```python
from build123d import *

# Parameters (mm, degrees)
CROQUIS1_R              = 11.5
CROQUIS1_R_2            = 4.35
CROQUIS1_R_3            = 1.7000000000000004
SALIENTE_EXTRUIR1_DEPTH = 3.5
CROQUIS2_R              = 5.35
CROQUIS2_R_2            = 4.35
SALIENTE_EXTRUIR2_DEPTH = 14
CORTAR_EXTRUIR1_START   = -5
CORTAR_EXTRUIR1_DEPTH   = 5
CROQUIS4_R              = 5.275
CROQUIS4_R_2            = 4.35
CORTAR_EXTRUIR2_DEPTH   = 2
REDONDEO1_R             = 0.6
REDONDEO2_R             = 0.5
SALIENTE_EXTRUIR3_DEPTH = 3.5


with BuildPart() as part:
    # Croquis1 → Saliente-Extruir1 (new body)
    with BuildSketch(Plane(origin=(0, 0, 0), x_dir=(1, 0, 0), z_dir=(0, 1, 0))):
        with Locations(Location((1.731948e-11, 0, 0), (0, 0, 270))):
            Circle(CROQUIS1_R)
        with Locations(Location((1.731948e-11, 0, 0), (0, 0, 270))):
            Circle(CROQUIS1_R_2, mode=Mode.SUBTRACT)
        with Locations(Location((5.656854249492441, 5.65685424949238, 0), (0, 0, 270))):
            Circle(CROQUIS1_R_3, mode=Mode.SUBTRACT)
        with Locations(Location((-5.656854249492318, 5.656854249492381, 0), (0, 0, 270))):
            Circle(CROQUIS1_R_3, mode=Mode.SUBTRACT)
        with Locations(Location((-5.656854249492318, -5.656854249492381, 0), (0, 0, 270))):
            Circle(CROQUIS1_R_3, mode=Mode.SUBTRACT)
        with Locations(Location((5.656854249492441, -5.65685424949238, 0), (0, 0, 270))):
            Circle(CROQUIS1_R_3, mode=Mode.SUBTRACT)
    extrude(amount=SALIENTE_EXTRUIR1_DEPTH)

    # Croquis2 → Saliente-Extruir2 (add)
    with BuildSketch(Plane(origin=(0, 3.5, 0), x_dir=(1, 0, 0), z_dir=(0, 1, 0))):
        with Locations(Location((1.731948e-11, 0, 0), (0, 0, 270))):
            Circle(CROQUIS2_R)
        with Locations(Location((1.731948e-11, 0, 0), (0, 0, 270))):
            Circle(CROQUIS2_R_2, mode=Mode.SUBTRACT)
    extrude(amount=SALIENTE_EXTRUIR2_DEPTH)

    # Croquis3 → Cortar-Extruir1 (cut)
    with BuildSketch(Plane(origin=(0, 17.5, 0), x_dir=(1, 0, 0), z_dir=(0, 1, 0)).offset(CORTAR_EXTRUIR1_START)):
        with BuildLine():
            Line((1.732086e-11, 5.35), (1.732072e-11, 4.35))
            ThreePointArc((1.732072e-11, 4.35), (3.0759144981543076, 3.0759144981369877), (4.34999999998268, 0))
            Line((4.34999999998268, 0), (5.34999999998268, 0))
            ThreePointArc((5.34999999998268, 0), (3.783021279340855, 3.783021279323535), (1.732086e-11, 5.35))
        make_face()
        with BuildLine():
            Line((1.732086e-11, -5.35), (1.732072e-11, -4.35))
            ThreePointArc((1.732072e-11, -4.35), (-3.075914498144163, -3.075914498161481), (-4.34999999998268, 0))
            Line((-4.34999999998268, 0), (-5.34999999998268, 0))
            ThreePointArc((-5.34999999998268, 0), (-3.7830212793307103, -3.7830212793480285), (1.732086e-11, -5.35))
        make_face()
    extrude(amount=CORTAR_EXTRUIR1_DEPTH, mode=Mode.SUBTRACT)

    # Croquis4 → Cortar-Extruir2 (cut)
    with BuildSketch(Plane.XZ):
        with Locations(Location((1.731948e-11, 0, 0), (0, 0, 270))):
            Circle(CROQUIS4_R)
        with Locations(Location((1.731948e-11, 0, 0), (0, 0, 270))):
            Circle(CROQUIS4_R_2, mode=Mode.SUBTRACT)
    extrude(amount=-CORTAR_EXTRUIR2_DEPTH, mode=Mode.SUBTRACT)

    # Redondeo1
    redondeo1_edges = [part.edges().sort_by_distance(p)[0] for p in [
        (1.732109e-11, 0, 5.275),
    ]]
    fillet(redondeo1_edges, radius=REDONDEO1_R)

    # Redondeo2
    # the kernel refuses this fillet: 0.5 mm, written as the material it takes off along each edge
    with BuildSketch(Plane(origin=(-4.34999999998268, 12.5, -2.1e-16), x_dir=(0.05161519234821224, 0, -0.9986670475783493), z_dir=(0, 1, 0))) as redondeo2_piece_1:
        with BuildLine():
            CenterArc((0.4748597696035476, 0.49933352378917434), REDONDEO2_R, 182.9586473758917, 84.08270524821648)
            Line((-0.02447375418562714, 0.4735259276150691), (0, 0))
            ThreePointArc((0, 0), (0.22452608671472166, 0.00579834303418057), (0.44905217342944187, 0))
        make_face()
    extrude(amount=6.185394894032285, mode=Mode.SUBTRACT)
    with BuildSketch(Plane(origin=(-5.34999999998268, 12.5, 0), x_dir=(1, 0, 0), z_dir=(0, 1, 0))) as redondeo2_piece_2:
        with BuildLine():
            CenterArc((0.5258420423870858, 0.5), REDONDEO2_R, 174.08270524821654, 95.91729475178346)
            ThreePointArc((0.02850617046822812, 0.5515463917525764), (0.00713129545583069, 0.27614127906293384), (0, 0))
            Line((0, 0), (0.5258420423870858, 0))
        make_face()
    extrude(amount=6.3807063953146645, mode=Mode.SUBTRACT)
    with BuildSketch(Plane(origin=(1.73185e-11, 12.5, 5.35), x_dir=(4.4e-15, 0, -1), z_dir=(0, 1, 0))) as redondeo2_piece_3:
        with BuildLine():
            CenterArc((0.5258420423870889, -0.5), REDONDEO2_R, 90.00000000000026, 95.91729475178363)
            ThreePointArc((0.02850617046823233, -0.5515463917525796), (0.0071312954558319, -0.27614127906293445), (0, 0))
            Line((0, 0), (0.5258420423870867, 0))
        make_face()
    extrude(amount=6.380706395314672, mode=Mode.SUBTRACT)
    with BuildSketch(Plane(origin=(1.731868e-11, 12.5, 4.35), x_dir=(0.9986670475783493, 0, -0.051615192348211894), z_dir=(0, 1, 0))) as redondeo2_piece_4:
        with BuildLine():
            CenterArc((0.474859769603551, -0.49933352378917434), REDONDEO2_R, 92.95864737589183, 84.08270524821639)
            Line((-0.0244737541856237, -0.4735259276150684), (0, 0))
            ThreePointArc((0, 0), (0.2245260867147224, -0.00579834303418053), (0.4490521734294448, 0))
        make_face()
    extrude(amount=6.185394894032285, mode=Mode.SUBTRACT)
    with BuildSketch(Plane(origin=(1.732072e-11, 12.5, -4.35), x_dir=(-0.9986670475783493, 0, 0.05161519234821218), z_dir=(0, 1, 0))) as redondeo2_piece_5:
        with BuildLine():
            CenterArc((0.474859769603548, -0.49933352378917434), REDONDEO2_R, 92.95864737589177, 84.08270524821641)
            Line((-0.02447375418562666, -0.47352592761506823), (0, 0))
            ThreePointArc((0, 0), (0.22452608671472019, -0.00579834303418048), (0.4490521734294423, 0))
        make_face()
    extrude(amount=6.185394894032285, mode=Mode.SUBTRACT)
    with BuildSketch(Plane(origin=(1.732103e-11, 12.5, -5.35), x_dir=(-4.2e-16, 0, 1), z_dir=(0, 1, 0))) as redondeo2_piece_6:
        with BuildLine():
            CenterArc((0.525842042387086, -0.5), REDONDEO2_R, 90.00000000000003, 95.91729475178352)
            ThreePointArc((0.02850617046822835, -0.5515463917525767), (0.00713129545583081, -0.27614127906293173), (0, 0))
            Line((0, 0), (0.5258420423870858, 0))
        make_face()
    extrude(amount=6.3807063953146645, mode=Mode.SUBTRACT)
    with BuildSketch(Plane(origin=(4.34999999998268, 12.5, 1.9e-16), x_dir=(-0.05161519227127975, 0, 0.9986670475823255), z_dir=(0, 1, 0))) as redondeo2_piece_7:
        with BuildLine():
            CenterArc((0.47485976964022647, 0.4993335237871862), REDONDEO2_R, 182.95864737147792, 84.08270524821648)
            Line((-0.02447375415093636, 0.4735259276515472), (0, 0))
            ThreePointArc((0, 0), (0.22452608671427532, 0.00579834305147695), (0.44905217342765447, 0))
        make_face()
    extrude(amount=6.1853948941188825, mode=Mode.SUBTRACT)
    with BuildSketch(Plane(origin=(5.34999999998268, 12.5, 0), x_dir=(-1, 0, 0), z_dir=(0, 1, 0))) as redondeo2_piece_8:
        with BuildLine():
            CenterArc((0.5258420423524468, 0.5), REDONDEO2_R, 174.08270524821646, 95.91729475178352)
            ThreePointArc((0.02850617043359005, 0.5515463917525769), (0.0071312954212388, 0.2761412790638265), (0, 0))
            Line((0, 0), (0.5258420423524468, 0))
        make_face()
    extrude(amount=6.380706395310195, mode=Mode.SUBTRACT)

    # Croquis5 → Saliente-Extruir3 (add)
    with BuildSketch(Plane(origin=(0, 3.5, 0), x_dir=(1, 0, 0), z_dir=(0, 1, 0))):
        with BuildLine():
            Line((-4.867801495370659, 2.219686599837588), (-10.46349854147086, 4.7712889529219185))
            ThreePointArc((-10.46349854147086, 4.7712889529219185), (-11.49999999998268, 1.41e-15), (-10.46349854147086, -4.771288952921916))
            Line((-10.46349854147086, -4.771288952921914), (-4.86780149537066, -2.219686599837586))
            ThreePointArc((-4.86780149537066, -2.219686599837586), (-5.34999999998268, 8.9e-16), (-4.86780149537066, 2.219686599837588))
        make_face()
        with BuildLine():
            Line((-2.2196865998351183, -4.867801495381207), (-4.77128895293652, -10.463498541473625))
            ThreePointArc((-4.771288952936522, -10.463498541473623), (-6.77758e-12, -11.5), (4.771288952927311, -10.463498541493617))
            Line((4.771288952927309, -10.46349854149362), (2.2196865998493576, -4.86780149539051))
            ThreePointArc((2.219686599849358, -4.867801495390509), (6.10956e-12, -5.35), (-2.219686599835118, -4.867801495381206))
        make_face()
        with BuildLine():
            ThreePointArc((11.50000000001732, 0), (11.237887551221265, 2.4412872396535783), (10.463498541496383, 4.771288952941911))
            Line((10.463498541496381, 4.7712889529419105), (4.867801495401058, 2.2196865998468893))
            ThreePointArc((4.867801495401059, 2.2196865998468898), (5.228060730360026, 1.1357292810562294), (5.350000000017321, -1.1e-16))
            ThreePointArc((5.350000000017321, -1.1e-16), (5.228060730360026, -1.1357292810562303), (4.867801495401057, -2.2196865998468898))
            Line((4.867801495401058, -2.2196865998468898), (10.463498541496381, -4.771288952941912))
            ThreePointArc((10.463498541496378, -4.7712889529419185), (11.237887551221265, -2.4412872396535787), (11.50000000001732, -2.82e-15))
        make_face()
        with BuildLine():
            ThreePointArc((4.771288952927309, 10.46349854149362), (-6.77732e-12, 11.5), (-4.771288952936519, 10.463498541473625))
            Line((-4.771288952936519, 10.463498541473623), (-2.2196865998351187, 4.867801495381207))
            ThreePointArc((-2.219686599835118, 4.867801495381207), (6.10867e-12, 5.35), (2.219686599849357, 4.86780149539051))
            Line((2.2196865998493576, 4.86780149539051), (4.771288952927309, 10.46349854149362))
        make_face()
    extrude(amount=SALIENTE_EXTRUIR3_DEPTH)


solid = part.part
```
Build history of the part. All positions in model axes, mm. A direction names the side the tool comes from. Coordinates: 2 decimals unless noted, no trailing zeros. Order: outer loops, then holes, each group sorted by start corner. A loop starts at its lowest first (then second) coordinate and runs counter-clockwise, first axis right, second up.
Item 1: Drill centre lines: L1, parallel to Y at x = 9.5, z = 1.5; L2, parallel to Y at x = 2, z = -4.75; L3, parallel to X at y = 5.5, z = -1.5. Where is each one in solid material? Low to high.
Filled in:
L1: y = 0 to 7
L2: y = 2 to 12.5
L3: x = -11.4 to -4.08, 4.08 to 11.4
Item 2: Mould opens along X. For faces 1 (the flat face through (3.51, 5.23, 7.7)), 2 (the flat face through (7, 3.5, -7)), 3 (the flat face through (-8, 0, 0)) say: released by +X, released by -X, zero draft, split by the parting line, or undercut.
Filled in:
face 1: released by +X
face 2: undercut
face 3: zero draft
Item 3: Saw through at B-B on x = 9.75. List the corners of the cut face in (y, z).
Filled in:
outline: (0, -6.1) - (3.5, -6.1) - (3.5, -4.45) - (7, -4.45) - (7, 4.45) - (3.5, 4.45) - (3.5, 6.1) - (0, 6.1) - close
Item 4: Drop flat-ended pins along their axis: pin 1 Ø5 at (x, y) = (2.5, 15) entering from +Z; pin 2 Ø2 at (x, z) = (-2.5, 7) entering from +Y; pin 3 Ø8.5 at (x, z) = (-1, -1) entering from -Y. Give the stop position or say it passes through.
Filled in:
pin 1: stops at z = 5.32
pin 2: stops at y = 7
pin 3: stops at y = 0.04
Item 5: Saw through at C-C on z = 9.5. List the corners of the cut face in (x, y), then the cut area to 3 significant figures.
Filled in:
outline: (-6.48, 0) - (6.48, 0) - (6.48, 3.5) - (4.33, 3.5) - (4.33, 7) - (-4.33, 7) - (-4.33, 3.5) - (-6.48, 3.5) - close
area: 75.7 mm2
Item 6: Saw through at D-D on y = 2.5. List the corners of the cut face in (x, z).
Filled in:
outline: circle Ø23 at (0, 0); hole circle Ø3.4 at (-5.66, -5.66); hole circle Ø3.4 at (-5.66, 5.66); hole circle Ø8.7 at (0, 0); hole circle Ø3.4 at (5.66, -5.66); hole circle Ø3.4 at (5.66, 5.66)
Item 7: Saw through at A-A on y = 6. List the corners of the cut face in (x, z).
Filled in:
outline: (-10.46, -4.77) - (-4.87, -2.22) arc R5.35 ccw to (-2.22, -4.87) - (-4.77, -10.46) arc R11.5 ccw to (4.77, -10.46) - (2.22, -4.87) arc R5.35 ccw to (4.87, -2.22) - (10.46, -4.77) arc R11.5 ccw to (10.46, 4.77) - (4.87, 2.22) arc R5.35 ccw to (2.22, 4.87) - (4.77, 10.46) arc R11.5 ccw to (-4.77, 10.46) - (-2.22, 4.87) arc R5.35 ccw to (-4.87, 2.22) - (-10.46, 4.77) arc R11.5 ccw to start; hole circle Ø8.7 at (0, 0)
Item 8: Tool access for faces 4 (the flat face through (-3.48, 5.23, 7.63)), 5 (the flat face through (7.7, 5.23, -3.51)), 6 (the cylindrical face through (3.565, 1.29, 3.888)), 7 (the flat face through (-7.7, 5.23, 3.51)): list every direction of +Z, -Z, +X, -X, +Y, -Y with a clear straight run to the whole face (end or side of a thin tool).
Filled in:
face 4: -X, +Y
face 5: -Z, +Y
face 6: -Y
face 7: +Z, +Y
